from build123d import *

# Parameters (mm, degrees)
SKETCH_1_R          = 1.4
EXTRUDE_1_DEPTH     = 8.2
CUT_EXTRUDE_1_DEPTH = 10
EXTRUDE_2_DEPTH     = 8.2
FILLET_1_R          = 2


with BuildPart() as part:
    # 草图1 → 凸台-拉伸1 (new body)
    with BuildSketch(Plane.XY):
        with BuildLine():
            Line((-13, 1), (-13, -12.307577498))
            ThreePointArc((-13, -12.307577498), (0, -7.8), (13, -12.307577498))
            Line((13, -12.307577498), (13, 1))
            ThreePointArc((13, 1), (12.121320344, 3.121320344), (10, 4))
            Line((10, 4), (-10, 4))
            ThreePointArc((-10, 4), (-12.121320344, 3.121320344), (-13, 1))
        make_face()
        with Locations((-9, 0)):
            Circle(SKETCH_1_R, mode=Mode.SUBTRACT)
        with Locations(Location((9, 0, 0), (0, 0, 180))):
            Circle(SKETCH_1_R, mode=Mode.SUBTRACT)
    extrude(amount=EXTRUDE_1_DEPTH)

    # 草图2 → 切除-拉伸1 (cut)
    with BuildSketch(Plane.XY.offset(8.2)):
        with BuildLine():
            ThreePointArc((-5, 0), (-7, -3.464101615), (-11, -3.464101615))
            Line((-11, -3.464101615), (-11, -8.600990123))
            ThreePointArc((-11, -8.600990123), (0, -5.8), (11, -8.600990123))
            Line((11, -8.600990123), (11, -3.464101615))
            ThreePointArc((11, -3.464101615), (7, -3.464101615), (5, 0))
            Line((5, 0), (-5, 0))
        make_face()
    extrude(amount=-CUT_EXTRUDE_1_DEPTH, mode=Mode.SUBTRACT)

    # 草图3 → 凸台-拉伸2 (add)
    with BuildSketch(Plane.XY.offset(8.2)):
        with BuildLine():
            Line((0, -5.8), (0, 0))
            Line((0, 0), (-1.5, 0))
            Line((-1.5, 0), (-1.5, -5.848965165))
            ThreePointArc((-1.5, -5.848965165), (-0.750399492, -5.812244551), (0, -5.8))
        make_face()
    extrude(amount=-EXTRUDE_2_DEPTH)

    # 圆角1
    # the kernel refuses this fillet: 2 mm, written as the material it adds along each edge
    with BuildSketch(Plane(origin=(-11, -8.600990123, 8.2), x_dir=(0, 1, 0), z_dir=(0, 0, -1))) as fillet_1_piece_1:
        with BuildLine():
            CenterArc((3.124797703, 2), FILLET_1_R, 158.899803976, 111.100196024)
            ThreePointArc((1.258893096, 2.72), (0.673800117, 1.339471911), (0, 0))
            Line((0, 0), (3.124797703, 0))
        make_face()
    extrude(amount=8.2)
    with BuildSketch(Plane(origin=(-11, -3.464101615, 8.2), x_dir=(0.9659258262890684, -0.2588190451025207, 0), z_dir=(0, 0, -1))) as fillet_1_piece_2:
        with BuildLine():
            CenterArc((2.588190451, 1.931851653), FILLET_1_R, 165, 90)
            Line((0.656338798, 2.449489743), (0, 0))
            ThreePointArc((0, 0), (1.03527618, 0.136296695), (2.070552361, 0))
        make_face()
    extrude(amount=8.2)
    with BuildSketch(Plane(origin=(-5, 0, 8.2), x_dir=(1, 0, 0), z_dir=(0, 0, -1))) as fillet_1_piece_3:
        with BuildLine():
            CenterArc((1.656854249, 2), FILLET_1_R, 199.471220634, 70.528779366)
            ThreePointArc((-0.228763834, 1.333333333), (-0.057605761, 0.676407915), (0, 0))
            Line((0, 0), (1.656854249, 0))
        make_face()
    extrude(amount=8.2)
    with BuildSketch(Plane(origin=(11, -3.464101615, 8.2), x_dir=(0, -1, 0), z_dir=(0, 0, -1))) as fillet_1_piece_4:
        with BuildLine():
            CenterArc((2.535898385, 2), FILLET_1_R, 180, 90)
            ThreePointArc((0.535898385, 2), (0.39960169, 0.96472382), (0, 0))
            Line((0, 0), (2.535898385, 0))
        make_face()
    extrude(amount=8.2)
    with BuildSketch(Plane(origin=(11, -8.600990123, 8.2), x_dir=(-0.9075134779972225, 0.42002296038833975, 0), z_dir=(0, 0, -1))) as fillet_1_piece_5:
        with BuildLine():
            CenterArc((3.127513738, 1.99575011), FILLET_1_R, 155.163962917, 111.100196024)
            Line((1.312486782, 2.835796031), (0, 0))
            ThreePointArc((0, 0), (1.498600333, 0.04887373), (2.997200665, 0))
        make_face()
    extrude(amount=8.2)
    with BuildSketch(Plane(origin=(5, 0, 8.2), x_dir=(-1, 0, 0), z_dir=(0, 0, -1))) as fillet_1_piece_6:
        with BuildLine():
            CenterArc((1.656854249, -2), FILLET_1_R, 90, 70.528779366)
            ThreePointArc((-0.228763834, -1.333333333), (-0.057605761, -0.676407915), (0, 0))
            Line((0, 0), (1.656854249, 0))
        make_face()
    extrude(amount=8.2)
    with BuildSketch(Plane(origin=(-1.5, 0, 8.2), x_dir=(-1, 0, 0), z_dir=(0, 0, -1))) as fillet_1_piece_7:
        with BuildLine():
            CenterArc((FILLET_1_R, -FILLET_1_R), FILLET_1_R, 90, 90)
            Line((0, -FILLET_1_R), (0, 0))
            Line((0, 0), (FILLET_1_R, 0))
        make_face()
    extrude(amount=8.2)
    with BuildSketch(Plane(origin=(-1.5, -5.848965165, 8.2), x_dir=(-0.994714309544396, -0.10268126600123115, 0), z_dir=(0, 0, -1))) as fillet_1_piece_8:
        with BuildLine():
            CenterArc((1.804319684, 1.998586493), FILLET_1_R, 185.893590739, 81.952153753)
            Line((-0.185108935, 1.793223961), (0, 0))
            ThreePointArc((0, 0), (0.864569849, 0.016255332), (1.729139697, 0))
        make_face()
    extrude(amount=8.2)
    with BuildSketch(Plane(origin=(0, -5.8, 8.2), x_dir=(0.9991983946019533, -0.04003208993893798, 0), z_dir=(0, 0, -1))) as fillet_1_piece_9:
        with BuildLine():
            CenterArc((1.921540317, -1.998396789), FILLET_1_R, 92.294282868, 85.411434264)
            Line((-0.076856472, -1.918332609), (0, 0))
            ThreePointArc((0, 0), (0.920738069, -0.018436924), (1.841476137, 0))
        make_face()
    extrude(amount=8.2)
    with BuildSketch(Plane(origin=(0, 0, 8.2), x_dir=(1, 0, 0), z_dir=(0, 0, -1))) as fillet_1_piece_10:
        with BuildLine():
            CenterArc((FILLET_1_R, FILLET_1_R), FILLET_1_R, 180, 90)
            Line((0, FILLET_1_R), (0, 0))
            Line((0, 0), (FILLET_1_R, 0))
        make_face()
    extrude(amount=8.2)
    # the kernel refuses this fillet: 2 mm, written as the material it takes off along each edge
    with BuildSketch(Plane(origin=(13, -12.307577498, -9.266468436), x_dir=(-0.8347589906571732, 0.5506154987984059, 0), z_dir=(0, 0, 1))) as fillet_1_2_piece_1:
        with BuildLine():
            CenterArc((3.710422437, -1.992876138), FILLET_1_R, 94.837370868, 118.571878142)
            Line((2.040904456, -3.094107135), (0, 0))
            ThreePointArc((0, 0), (1.770883436, -0.074800554), (3.541766872, 0))
        make_face()
    extrude(amount=26.732936871, mode=Mode.SUBTRACT)
    with BuildSketch(Plane(origin=(-13, -12.307577498, -9.266468436), x_dir=(0, 1, 0), z_dir=(0, 0, 1))) as fillet_1_2_piece_2:
        with BuildLine():
            CenterArc((3.706587374, -2), FILLET_1_R, 90, 118.571878142)
            ThreePointArc((1.950151733, -2.956521739), (1.037516301, -1.437074525), (0, 0))
            Line((0, 0), (3.706587374, 0))
        make_face()
    extrude(amount=26.732936871, mode=Mode.SUBTRACT)


solid = part.part
Could you check a few things on this model? Use its own coordinates, in mm. A direction names the side the tool comes from. Give positions to 0.01 mm unless a question says otherwise; leave off trailing zeros. Loops run counter-clockwise (first coordinate to the right, second up) from the corner with the lowest first, then second, coordinate; pieces in that order, holes last. Notation, with made-up numbers: (-8.75, -0.5) -> (6.25, -0.5) arc R28 ccw to (6.25, 22.5) -> close; hole circle Ø9 at (74, 85). An arc over 180 degrees is marked (long way). Return JSON: item names as keys, results as strings.
Item 1: I'm going to push flat-ended pins straight in: pin 1 (5 mm diameter, centred on x = -8, y = -3, fed in from -Z); pin 2 (2.5 mm diameter, centred on x = -9, y = 0, fed in from -Z) (3 decimals); pin 3 (1.5 mm diameter, centred on x = 2.5, z = 5.5, fed in from -Y). Where does each tip first touch, or does it pass through?
Geometry results:
{"pin 1": "stops at z = 0", "pin 2": "passes through", "pin 3": "stops at y = -8.05"}
Item 2: I need wall thicknesses on L1, parallel to X at y = 1.25, z = 4.75; L2, parallel to Y at x = 9, z = 5.25; L3, parallel to Y at x = -7.75, z = 4.75. Which ranges of each line are inside material? Lowest first, please. Write a range as from..to.
Geometry results:
{"L1": "x = -12.99..-9.63, -8.37..8.37, 9.63..12.99", "L2": "y = -9.83..-7.48, -4..-1.4, 1.4..4", "L3": "y = -9.28..-7.15, -3.8..-0.63, 0.63..4"}
Item 3: Which directions (+Z, -Z, +X, -X, +Y, -Y) give clear straight access to the entire face, cutting with the end or side of a thin tool? Please do faces 4 (the cylindrical face through (-10, -7.21, 4.16)), 5 (the flat face through (0, 4, 4)).
Geometry results:
{"face 4": "+Z, -Z", "face 5": "+Z, -Z, +X, -X, +Y"}
Item 4: If we section it at B-B on y = -4.5: List the corners of the cut face in (x, z) for me.
Geometry results:
{"outline": "(-13, 0) -> (-10.32, 0) -> (-10.32, 8.2) -> (-13, 8.2) -> close; (-1.55, 0) -> (0.1, 0) -> (0.1, 8.2) -> (-1.55, 8.2) -> close; (10.32, 0) -> (13, 0) -> (13, 8.2) -> (10.32, 8.2) -> close"}
Item 5: If we section it at A-A on z = 6: List the corners of the cut face in (x, y) for me, plus the area to 3 significant figures.
Geometry results:
{"outline": "(-13, -8.6) arc R2 ccw to (-10.04, -10.36) arc R21 cw to (10.04, -10.36) arc R2 ccw to (13, -8.6) -> (13, 1) arc R3 ccw to (10, 4) -> (-10, 4) arc R3 ccw to (-13, 1) -> close; hole (-10.98, -5.74) arc R2 ccw to (-8.28, -7.34) arc R23 cw to (-3.22, -6.03) arc R2 ccw to (-1.5, -4.05) -> (-1.5, -2) arc R2 ccw to (-3.42, 0) arc R2 ccw to (-5.23, -1.33) arc R4 cw to (-9, -4) arc R2 ccw to start; hole circle Ø2.8 at (-9, 0); hole (0, -3.88) arc R2 ccw to (1.84, -5.87) arc R23 cw to (8.28, -7.34) arc R2 ccw to (10.98, -5.74) arc R2 ccw to (9, -4) arc R4 cw to (5.23, -1.33) arc R2 ccw to (3.34, 0) -> (2, 0) arc R2 ccw to (0, -2) -> close; hole circle Ø2.8 at (9, 0)", "area": "234 mm²"}
Item 6: We'd pull the mould along Y, two halves only. Please class faces 1 (the flat face through (13, -4, 4)), 2 (the flat face through (-1.5, -3, 4)), 3 (the cylindrical face through (12.14, 3.1, 4.04)): +Y half, -Y half, draft (parallel to the pull), parting line (faces both ways), or undercut.
Geometry results:
{"face 1": "draft", "face 2": "undercut", "face 3": "+Y half"}
